The drawing under review shows one solid part. Ordinate dimensions are in mm from its lowest x, y, z. Coordinates: 2 decimals unless noted, no trailing zeros. Loops run counter-clockwise (first coordinate to the right, second up) from the corner with the lowest first, then second, coordinate; pieces in that order, holes last. Notation, with made-up numbers: M -20,-38 L 16,-38 A14 ccw 16,-27 Z; hole C 62.5,20 d10. An arc over 180 degrees is marked long. Answer as a JSON object with one key per item and string values. Group by question number.
1. Consider section D-D (y = 3). State the section outline as (x, z) points.
2. Consider section A-A (y = 20). State the section outline as (x, z) points (1 decimal).
3. Draft analysis for pull direction Y (two halves, no side actions). For the marked faces 1, 2, 3 and 4, state which applies: +Y half, -Y half, draft (parallel to the pull), parting line (faces both ways), or undercut.
4. Consider section B-B (z = 12). State the section outline as (x, y) points.
5. Insertion check: pin 1 (2 mm diameter, centred on x = 6, z = 40.5, fed in from -Y); pin 2 (10 mm diameter, centred on x = 22, y = 29, fed in from -Z); pin 3 (2 mm diameter, centred on x = 5, z = 42, fed in from -Y). Each pin has a flat end and moves straight along its axis. Give the tip position at first contact, or say it passes through.
6. To check wall thickness, follow probe 1 along Z at (x, y) = (5, 22.5) (1 decimal); probe 2 along Z at (x, y) = (20.25, 22); probe 3 along Y at (x, z) = (7.5, 9). State the ranges of each line that lie inside material, in increasing order.
7. Consider section C-C (x = 3.25). State the section outline as (y, z) points.
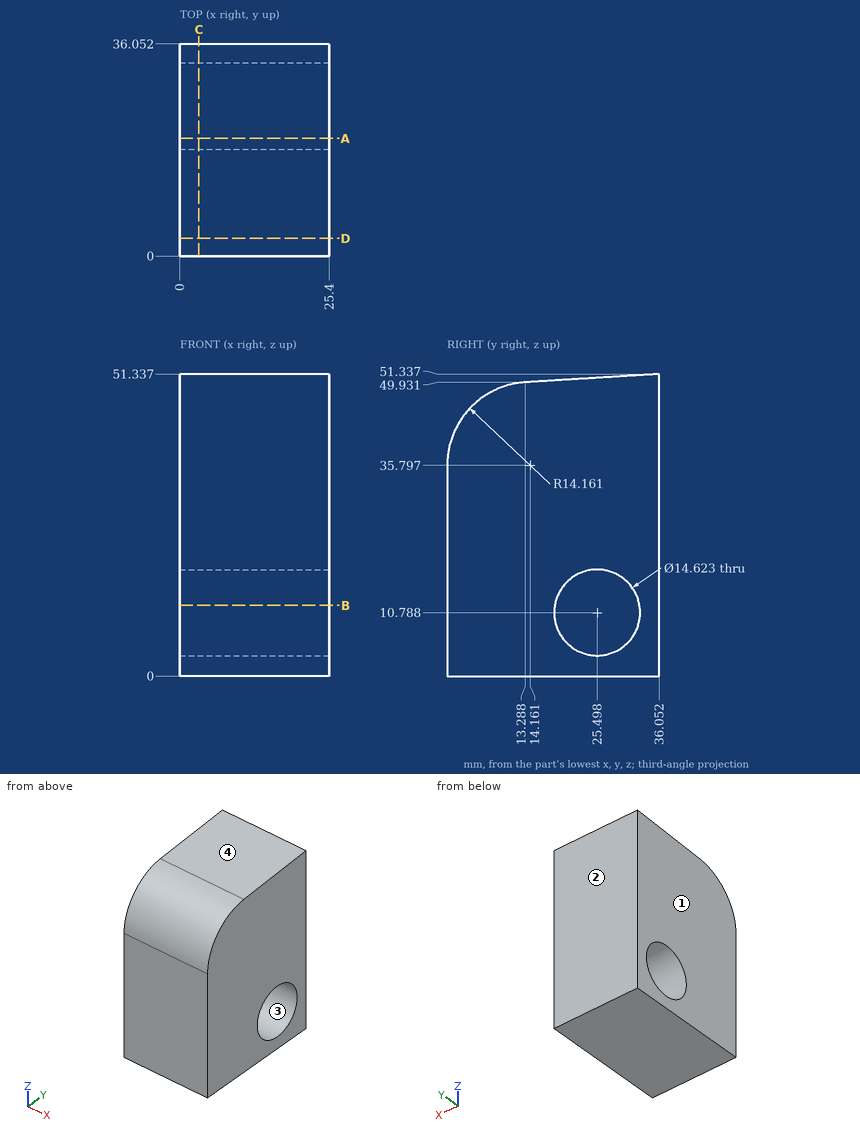
Findings below:
{
 "1": {"outline": "M 0,0 L 25.4,0 L 25.4,44.51 L 0,44.51 Z"},
 "2": {"outline": "M 0,0 L 25.4,0 L 25.4,6 L 0,6 Z; M 0,15.6 L 25.4,15.6 L 25.4,50.3 L 0,50.3 Z"},
 "3": {"face 1": "draft", "face 2": "+Y half", "face 3": "undercut", "face 4": "-Y half"},
 "4": {"outline": "M 0,0 L 25.4,0 L 25.4,18.29 L 0,18.29 Z; M 0,32.71 L 25.4,32.71 L 25.4,36.05 L 0,36.05 Z"},
 "5": {"pin 1": "stops at y = 0.49", "pin 2": "stops at z = 0", "pin 3": "stops at y = 0.99"},
 "6": {"probe 1": "z = 0 to 4.1, 17.5 to 50.5", "probe 2": "z = 0 to 4.37, 17.21 to 50.47", "probe 3": "y = 0 to 18.41, 32.59 to 36.05"},
 "7": {"outline": "M 0,0 L 36.05,0 L 36.05,51.34 L 13.29,49.93 A14.16 ccw 0,35.8 Z; hole C 25.5,10.79 d14.62"}
}
